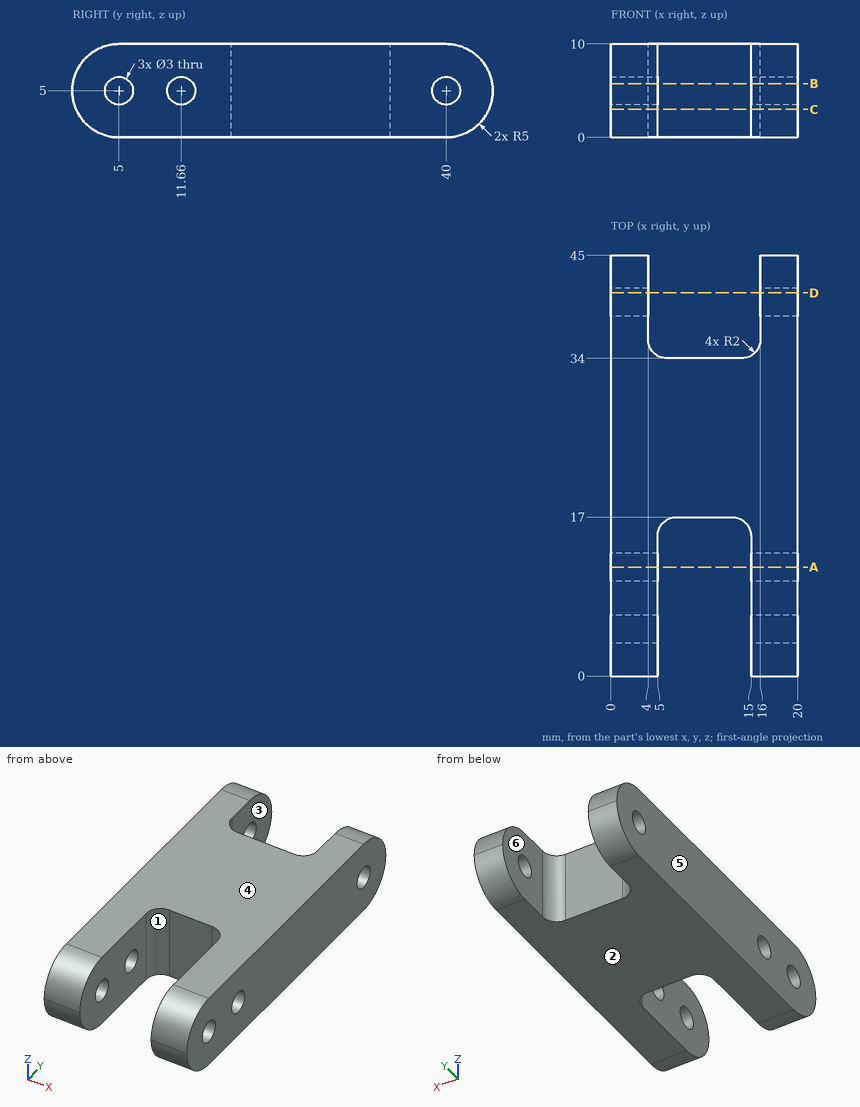
The figure shows three views and two pictorial views of one solid part (mm, origin at its lowest corner). Answer the questions. A direction names the side the tool comes from. Round coordinates to 2 decimals unless told otherwise and drop trailing zeros. Order: outer loops, then holes, each group sorted by start corner. A loop starts at its lowest first (then second) coordinate and runs counter-clockwise, first axis right, second up.
Q1. A cutting plane is placed at A-A, the plane y = 11.66. Determine the outline of the cut face in (x, z), then the cut area to 3 significant figures.
Solution:
outline: (0, 0) - (5, 0) - (5, 3.5) - (0, 3.5) - close; (0, 6.5) - (5, 6.5) - (5, 10) - (0, 10) - close; (15, 0) - (20, 0) - (20, 3.5) - (15, 3.5) - close; (15, 6.5) - (20, 6.5) - (20, 10) - (15, 10) - close
area: 70.0 mm2
Q2. A cutting plane is placed at B-B, the plane z = 5.75. Count the separate pieces of the cut face and the enclosed holes in it, then the cut area to 3 significant figures.
Solution:
separate pieces: 7
enclosed holes: 0
area: 528 mm2
Q3. A cutting plane is placed at C-C, the plane z = 3. Determine the outline of the cut face in (x, y).
Solution:
outline: (0, 0.42) - (5, 0.42) - (5, 15) arc R2 cw to (7, 17) - (13, 17) arc R2 cw to (15, 15) - (15, 0.42) - (20, 0.42) - (20, 44.58) - (16, 44.58) - (16, 36) arc R2 cw to (14, 34) - (6, 34) arc R2 cw to (4, 36) - (4, 44.58) - (0, 44.58) - close
Q4. The mould has two halves that part along X. Classify the marked faces 4, 5 and 6: pulls with the +X half, pulls with the -X half, needs draft (parallel to the pull), parting line crosses it, or undercut.
Solution:
face 4: needs draft
face 5: pulls with the -X half
face 6: undercut
Q5. Given pin 1 Ø2.5 at (y, z) = (5, 5) entering from +X; pin 2 Ø1 at (x, z) = (8.5, 6.5) entering from -Y, each flat-ended and moving along its own axis, determine where each tip first touches the part or whether it passes through.
Solution:
pin 1: passes through
pin 2: stops at y = 17
Q6. A cutting plane is placed at D-D, the plane y = 41. Determine the outline of the cut face in (x, z), then the cut area to 3 significant figures.
Solution:
outline: (0, 0.1) - (4, 0.1) - (4, 3.88) - (0, 3.88) - close; (0, 6.12) - (4, 6.12) - (4, 9.9) - (0, 9.9) - close; (16, 0.1) - (20, 0.1) - (20, 3.88) - (16, 3.88) - close; (16, 6.12) - (20, 6.12) - (20, 9.9) - (16, 9.9) - close
area: 60.5 mm2
Q7. Find the intervals of material crossed by line 1 along Y through (x, z) = (16.7, 5); line 2 along X through (y, z) = (39.5, 2); line 3 along Y through (x, z) = (2.25, 4), in increasing order.
Solution:
line 1: y = 0 to 3.5, 6.5 to 10.16, 13.16 to 38.5, 41.5 to 45
line 2: x = 0 to 4, 16 to 20
line 3: y = 0.1 to 3.88, 6.12 to 10.54, 12.78 to 38.88, 41.12 to 44.9
Q8. A tool of negligible diameter and unlimited length cuts with its end or side. For the marked faces 1, 2 and 3, from which of +Z, -Z, +X, -X, +Y, -Y can it reach the whole face along a straight path? Write none if from no direction.
Solution:
face 1: +Z, -Z, -Y
face 2: -Z, +X, -X, +Y, -Y
face 3: +Z, -Z, +Y
